Build history of the part. All positions in model axes, mm. Round coordinates to 2 decimals unless told otherwise and drop trailing zeros. Order: outer loops, then holes, each group sorted by start corner. A loop starts at its lowest first (then second) coordinate and runs counter-clockwise, first axis right, second up. Notation, with made-up numbers: (79.5, 11.25) -> (95.5, 11.25) arc R25 ccw to (95.5, 48.25) -> close; hole circle Ø8 at (67, 45). An arc over 180 degrees is marked (long way). Answer as CSV lines item,"result". Start each with the question number.
```python
from build123d import *

# Parameters (mm, degrees)
ESQUISSE1_R                                        = 5
BOSS_EXTRU_1_DEPTH                                 = 10
ESQUISSE2_R                                        = 11
ENL_V_MAT_EXTRU_1_DEPTH                            = 2
CHAMBRAGE_POUR_VIS_T_TE_HEXAGONALE_M41_D           = 4.5
CHAMBRAGE_POUR_VIS_T_TE_HEXAGONALE_M41_CBORE_D     = 8
CHAMBRAGE_POUR_VIS_T_TE_HEXAGONALE_M41_CBORE_DEPTH = 4.4
R_P_TITION_CIRCULAIRE1_COUNT                       = 4
CHAMBRAGE_POUR_VIS_T_TE_HEXAGONALE_M42_D           = 4.5
CHAMBRAGE_POUR_VIS_T_TE_HEXAGONALE_M42_CBORE_D     = 8
CHAMBRAGE_POUR_VIS_T_TE_HEXAGONALE_M42_CBORE_DEPTH = 4.4
CHAMBRAGE_POUR_VIS_T_TE_HEXAGONALE_M43_D           = 4.5
CHAMBRAGE_POUR_VIS_T_TE_HEXAGONALE_M43_CBORE_D     = 8
CHAMBRAGE_POUR_VIS_T_TE_HEXAGONALE_M43_CBORE_DEPTH = 4.4
R_P_TITION_CIRCULAIRE2_COUNT                       = 4
R_P_TITION_CIRCULAIRE3_COUNT                       = 4


with BuildPart() as part:
    # Esquisse1 → Boss.-Extru.1 (new body)
    with BuildSketch(Plane(origin=(0, 0, 0), x_dir=(1, 0, 0), z_dir=(0, 1, 0))):
        with BuildLine():
            Line((350, 0), (-350, 0))
            Line((-350, 0), (-350, 198.324835183))
            ThreePointArc((-350, 198.324835183), (-348.317239297, 203.876729496), (-343.835293906, 207.560121895))
            Line((-343.835293906, 207.560121895), (-47.941173826, 330.441083901))
            ThreePointArc((-47.941173826, 330.441083901), (0, 340), (47.941173826, 330.441083901))
            Line((47.941173826, 330.441083901), (343.835293906, 207.560121895))
            ThreePointArc((343.835293906, 207.560121895), (348.317239297, 203.876729496), (350, 198.324835183))
            Line((350, 198.324835183), (350, 0))
        make_face()
        with Locations(Location((0, 215, 0), (0, 0, 270))):
            Circle(ESQUISSE1_R, mode=Mode.SUBTRACT)
        with Locations(Location((-225, 125, 0), (0, 0, 270))):
            Circle(ESQUISSE1_R, mode=Mode.SUBTRACT)
        with Locations(Location((225, 125, 0), (0, 0, 90))):
            Circle(ESQUISSE1_R, mode=Mode.SUBTRACT)
    extrude(amount=BOSS_EXTRU_1_DEPTH)

    # Esquisse2 → Enl_v. mat.-Extru.1 (cut)
    with BuildSketch(Plane(origin=(0, 10, 0), x_dir=(1, 0, 0), z_dir=(0, 1, 0))):
        with Locations(Location((0, 215, 0), (0, 0, 270))):
            Circle(ESQUISSE2_R)
        with Locations(Location((225, 125, 0), (0, 0, 270))):
            Circle(ESQUISSE2_R)
        with Locations(Location((-225, 125, 0), (0, 0, 270))):
            Circle(ESQUISSE2_R)
    extrude(amount=-ENL_V_MAT_EXTRU_1_DEPTH, mode=Mode.SUBTRACT)

    # Chambrage pour vis _ t_te hexagonale M41 (through all)
    with Locations(Plane(origin=(0, 0, 0), x_dir=(-1, 0, 0), z_dir=(0, -1, 0))):
        with Locations((-225, 141)):
            chambrage_pour_vis_t_te_hexagonale_m41 = CounterBoreHole(CHAMBRAGE_POUR_VIS_T_TE_HEXAGONALE_M41_D / 2, CHAMBRAGE_POUR_VIS_T_TE_HEXAGONALE_M41_CBORE_D / 2, CHAMBRAGE_POUR_VIS_T_TE_HEXAGONALE_M41_CBORE_DEPTH)

    # R_p_tition circulaire1: Chambrage pour vis _ t_te hexagonale M41 ×4 about axis
    r_p_tition_circulaire1_axis = Axis((225, 0, -125), (0, 1, 0))
    for i in range(1, R_P_TITION_CIRCULAIRE1_COUNT):
        add(chambrage_pour_vis_t_te_hexagonale_m41.rotate(r_p_tition_circulaire1_axis, i * 360 / R_P_TITION_CIRCULAIRE1_COUNT), mode=Mode.SUBTRACT)

    # Chambrage pour vis _ t_te hexagonale M42 (through all)
    with Locations(Plane(origin=(0, 0, 0), x_dir=(-1, 0, 0), z_dir=(0, -1, 0))):
        with Locations((0, 231)):
            chambrage_pour_vis_t_te_hexagonale_m42 = CounterBoreHole(CHAMBRAGE_POUR_VIS_T_TE_HEXAGONALE_M42_D / 2, CHAMBRAGE_POUR_VIS_T_TE_HEXAGONALE_M42_CBORE_D / 2, CHAMBRAGE_POUR_VIS_T_TE_HEXAGONALE_M42_CBORE_DEPTH)

    # Chambrage pour vis _ t_te hexagonale M43 (through all)
    with Locations(Plane(origin=(0, 0, 0), x_dir=(-1, 0, 0), z_dir=(0, -1, 0))):
        with Locations((225, 141)):
            chambrage_pour_vis_t_te_hexagonale_m43 = CounterBoreHole(CHAMBRAGE_POUR_VIS_T_TE_HEXAGONALE_M43_D / 2, CHAMBRAGE_POUR_VIS_T_TE_HEXAGONALE_M43_CBORE_D / 2, CHAMBRAGE_POUR_VIS_T_TE_HEXAGONALE_M43_CBORE_DEPTH)

    # R_p_tition circulaire2: Chambrage pour vis _ t_te hexagonale M42 ×4 about axis
    r_p_tition_circulaire2_axis = Axis((0, 0, -215), (0, 1, 0))
    for i in range(1, R_P_TITION_CIRCULAIRE2_COUNT):
        add(chambrage_pour_vis_t_te_hexagonale_m42.rotate(r_p_tition_circulaire2_axis, i * 360 / R_P_TITION_CIRCULAIRE2_COUNT), mode=Mode.SUBTRACT)

    # R_p_tition circulaire3: Chambrage pour vis _ t_te hexagonale M43 ×4 about axis
    r_p_tition_circulaire3_axis = Axis((-225, 0, -125), (0, 1, 0))
    for i in range(1, R_P_TITION_CIRCULAIRE3_COUNT):
        add(chambrage_pour_vis_t_te_hexagonale_m43.rotate(r_p_tition_circulaire3_axis, i * 360 / R_P_TITION_CIRCULAIRE3_COUNT), mode=Mode.SUBTRACT)


solid = part.part
```
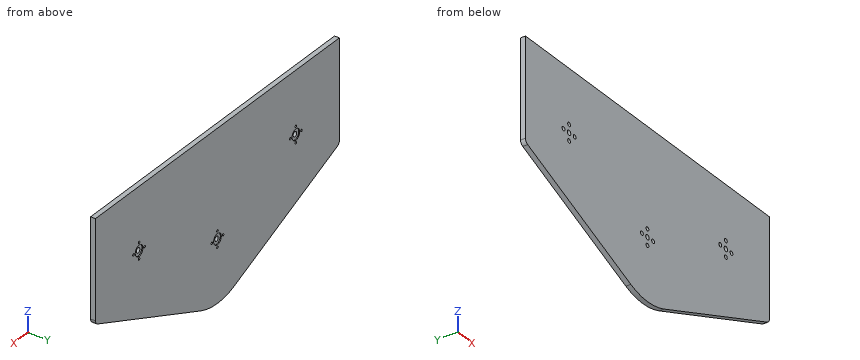
Q1. Probe L1, parallel to Z at x = 0, y = 5.6; L2, parallel to X at y = 9.25, z = -133.5; L3, parallel to X at y = 8.45, z = -199. List the from-to ranges inside material, lowest first.
Q2. Slice it at A-A, the plane y = 6.25. Count the separate pieces of the cut face and the enclosed holes in it, plus the area to 3 significant figures.
Q3. Slice it at C-C, the plane z = -289.5. Write the cut outline in (x, y), plus the area to 3 significant figures.
Q4. Slice it at B-B, the plane x = 126.5. Write the cut outline in (y, z).
Q5. Flat gauge pins, fed straight in: pin 1 Ø5 at (x, z) = (-225, -109) entering from -Y; pin 2 Ø5 at (y, z) = (3, -257.5) entering from +X; pin 3 Ø4 at (y, z) = (7, -285.5) entering from +X; pin 4 Ø3.5 at (x, z) = (209, -125) entering from -Y. Where does each tip first touch, or does it go through?
Solutions:
1,L1,"z = -340 to -233.25, -228.75 to -220, -210 to -201.25, -196.75 to 0"
1,L2,"x = -350 to -231.98, -218.02 to 218.02, 231.98 to 350"
1,L3,"x = -349.98 to -2.25, 2.25 to 349.98"
2,separate pieces,"1"
2,enclosed holes,"15"
2,area,"194,000 mm2"
3,outline,"(-146.53, 0) -> (146.53, 0) -> (146.53, 10) -> (-146.53, 10) -> close"
3,area,"2,930 mm2"
4,outline,"(0, -297.82) -> (10, -297.82) -> (10, 0) -> (0, 0) -> close"
5,pin 1,"stops at y = 4.4"
5,pin 2,"stops at x = 229.6"
5,pin 3,"stops at x = 160.97"
5,pin 4,"passes through"
